```python
from build123d import *

# Parameters (mm, degrees)
SKETCH1_R           = 9
BOSS_EXTRUDE1_DEPTH = 7
SKETCH2_R           = 5.5
CUT_EXTRUDE1_DEPTH  = 5
CHAMFER1_SIZE       = 1
CHAMFER1_SIZE2      = 5.144554016


with BuildPart() as part:
    # Sketch1 → Boss-Extrude1 (new body)
    with BuildSketch(Plane.XY):
        Circle(SKETCH1_R)
    extrude(amount=BOSS_EXTRUDE1_DEPTH)

    # Sketch2 → Cut-Extrude1 (cut)
    with BuildSketch(Plane.XY.offset(7)):
        Circle(SKETCH2_R)
    extrude(amount=-CUT_EXTRUDE1_DEPTH, mode=Mode.SUBTRACT)

    # Chamfer1
    chamfer1_edges = [part.edges().sort_by_distance(p)[0] for p in [
        (-9, 0, 7),
    ]]
    chamfer1_side = [part.faces().sort_by_distance(p)[0] for p in [
        (-8.745441559, 0, 7),
    ]]
    chamfer(chamfer1_edges, length=CHAMFER1_SIZE, length2=CHAMFER1_SIZE2, reference=chamfer1_side[0])


solid = part.part
```
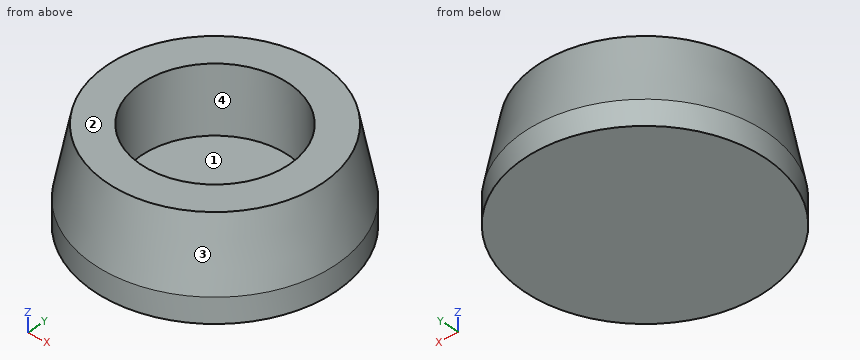
Source: CAD feature listing. Evaluate the final solid. Frame: model axes, mm. Face numbers are marked on the shaded views. Coordinates: 2 decimals unless noted, no trailing zeros. Write each loop counter-clockwise with the first axis right and the second up, starting at its lowest first coordinate (ties: lowest second). Pieces come first, ordered by that corner, then holes. Notation, with made-up numbers: M 8,-32 L 67,-32 A24 ccw 67,-1 Z; hole C -35.75,15.25 d5. An arc over 180 degrees is marked long. Answer as a JSON object with one key per item and string values.
1. Ray query, L1, parallel to Y at x = 0, z = 5.45; L2, parallel to X at y = 0.5, z = 3.5; L3, parallel to Y at x = 0, z = 4.1. Return the intervals inside material, ascending.
Evaluation:
{"L1": "-8.3 to -5.5, 5.5 to 8.3", "L2": "-8.67 to -5.48, 5.48 to 8.67", "L3": "-8.56 to -5.5, 5.5 to 8.56"}
2. Contact query for flat-ended pins moving along their axis: P1, Ø5.5, axis at x = 0, y = 2, coming from the +Z side; P2, Ø1, axis at x = -2.5, z = 5.5, coming from the -Y side; P3, Ø1, axis at x = -1, z = 4.5, coming from the -Y side; P4, Ø4, axis at x = -6.5, y = 5.5, coming from the +Z side. Output: stop coordinate, or through.
Evaluation:
{"P1": "z = 2", "P2": "y = -8.08", "P3": "y = -8.54", "P4": "z = 7"}
3. Draft query along Y for the marked faces 1, 2, 3 and 4. Return one class per face: released by +Y, released by -Y, zero draft, split by the parting line, or undercut.
Evaluation:
{"face 1": "undercut", "face 2": "zero draft", "face 3": "split by the parting line", "face 4": "undercut"}
4. Cut plane A-A on x = 0. Output: boundary loops of the cut face in (y, z).
Evaluation:
{"outline": "M -9,0 L 9,0 L 9,1.86 L 8,7 L 5.5,7 L 5.5,2 L -5.5,2 L -5.5,7 L -8,7 L -9,1.86 Z"}
5. Cut plane C-C on z = 1. Output: boundary loops of the cut face in (x, y).
Evaluation:
{"outline": "C 0,0 d18"}
6. Cut plane D-D on z = 5. Output: boundary loops of the cut face in (x, y), plus the area to 3 significant figures.
Evaluation:
{"outline": "C 0,0 d16.78; hole C 0,0 d11", "area": "126 mm^2"}
